For this review, take the finished solid that the model builds, in its own axes (mm). Coordinates: 2 decimals unless noted, no trailing zeros. Order: outer loops, then holes, each group sorted by start corner. A loop starts at its lowest first (then second) coordinate and runs counter-clockwise, first axis right, second up. Notation, with made-up numbers: (-2, -12) -> (51, -12) arc R13 ccw to (51, 8) -> close; hole circle Ø8 at (3.5, 57). An arc over 180 degrees is marked (long way). Write item = value, one per line. Start each with the question number.
1) Insertion check: pin 1 Ø6.5 at (x, z) = (0, 666.75) entering from -Y; pin 2 Ø3 at (y, z) = (5, -249.5) entering from -X; pin 3 Ø5 at (x, z) = (0, 30) entering from -Y; pin 4 Ø5 at (x, z) = (-7.5, -343.5) entering from -Y. Each pin has a flat end and moves straight along its axis. Give the tip position at first contact, or say it passes through.
2) Wall thickness on probe 1 along Z at (x, y) = (0, -12.05); probe 2 along Y at (x, z) = (1.75, 98.5); probe 3 along X at (y, z) = (-2, 296): over which ranges is each line inside the solid? List them lowest first. Write a range as [from, to].
3) Consider section A-A on y = 0. Give the boundary of the cut face in (x, z), and give its area (3 significant figures).
4) Consider section B-B on z = -119. Give the boundary of the cut face in (x, y) (1 decimal), and give its area (3 significant figures).
from build123d import *

# Parameters (mm, degrees)
SKETCH1_R                                  = 12.7
SKETCH1_R_2                                = 11.1125
BOSS_EXTRUDE1_DEPTH                        = 716.7546056
M5_CLEARANCE_HOLE1_D                       = 5.5
SKETCH7_W                                  = 2.75
SKETCH7_H                                  = 12.7
MIRROR1_AT_THE_SECOND_PLANE_COPY_1_SKETC_W = 2.75
MIRROR1_AT_THE_SECOND_PLANE_COPY_1_SKETC_H = 12.7
CUT_EXTRUDE1_START                         = -12.7
SKETCH8_R                                  = 2.5
CUT_EXTRUDE1_DEPTH                         = 25.4


with BuildPart() as part:
    # Sketch1 → Boss-Extrude1 (new body, symmetric)
    with BuildSketch(Plane.XY):
        Circle(SKETCH1_R)
        Circle(SKETCH1_R_2, mode=Mode.SUBTRACT)
    extrude(amount=BOSS_EXTRUDE1_DEPTH, both=True)

    # M5 Clearance Hole1 (through all)
    with Locations(Plane(origin=(0, 12.7, 0), x_dir=(1, 0, 0), z_dir=(0, 1, 0))):
        with Locations((0, 30), (0, -30)):
            Hole(M5_CLEARANCE_HOLE1_D / 2)

    # Sketch7 → M5 Clearance Hole2 (revolve, cut)
    with BuildSketch(Plane(origin=(0, 0, 666.7546056), x_dir=(0, 0, -1), z_dir=(1, 0, 0))):
        with Locations((1.375, 6.35)):
            Rectangle(SKETCH7_W, SKETCH7_H)
    m5_clearance_hole2 = revolve(axis=Axis((0, -6.35, 666.7546056), (0, 1, 0)), mode=Mode.SUBTRACT)

    # Mirror1: M5 Clearance Hole2 across plane
    add(m5_clearance_hole2.mirror(Plane.ZX), mode=Mode.SUBTRACT)

    # Mirror1 at the second plane: M5 Clearance Hole2 across plane
    add(m5_clearance_hole2.mirror(Plane.XY), mode=Mode.SUBTRACT)

    # Mirror1 at the second plane copy 1 sketc → Mirror1 at the second plane copy 1 (revolve, cut)
    with BuildSketch(Plane(origin=(0, 0, -666.7546056), x_dir=(0, 0, 1), z_dir=(1, 0, 0))):
        with Locations((1.375, 6.35)):
            Rectangle(MIRROR1_AT_THE_SECOND_PLANE_COPY_1_SKETC_W, MIRROR1_AT_THE_SECOND_PLANE_COPY_1_SKETC_H)
    revolve(axis=Axis((0, 6.35, -666.7546056), (0, -1, 0)), mode=Mode.SUBTRACT)

    # Sketch8 → Cut-Extrude1 (cut)
    with BuildSketch(Plane(origin=(0, 0, 0), x_dir=(-0.834407926, -0.55114736, 0), z_dir=(0.55114736, -0.834407926, 0)).offset(CUT_EXTRUDE1_START)):
        with Locations((1.717033262, 267.917598195)):
            Circle(SKETCH8_R)
    cut_extrude1 = extrude(amount=CUT_EXTRUDE1_DEPTH, mode=Mode.SUBTRACT)

    # Mirror2: Cut-Extrude1 across plane
    add(cut_extrude1.mirror(Plane.XY), mode=Mode.SUBTRACT)


solid = part.part
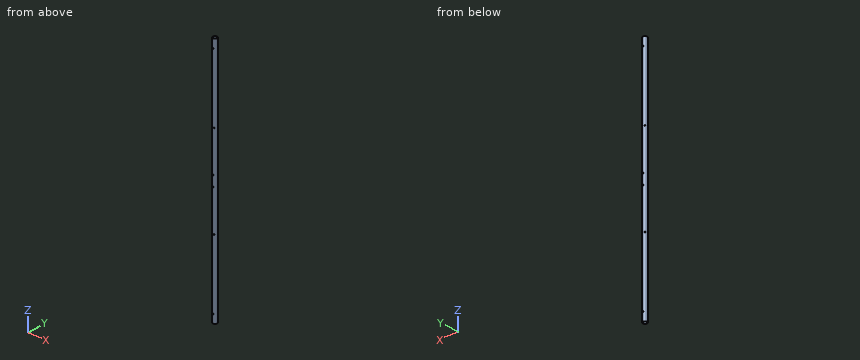
Answer sheet:
q1.pin_1 = -12.7
q1.pin_2 = -12.21
q1.pin_3 = through
q1.pin_4 = -11.67
q2.probe_1 = [-716.75, -669.5], [-664, -32.75], [-27.25, 27.25], [32.75, 664], [669.5, 716.75]
q2.probe_2 = [-12.58, -10.97], [10.97, 12.58]
q2.probe_3 = [-12.54, -10.93], [10.93, 12.54]
q3.outline = (-12.7, -716.75) -> (-11.11, -716.75) -> (-11.11, 716.75) -> (-12.7, 716.75) -> close; (11.11, -716.75) -> (12.7, -716.75) -> (12.7, 716.75) -> (11.11, 716.75) -> close
q3.area = 4,550 mm2
q4.outline = circle Ø25.4 at (0, 0); hole circle Ø22.2 at (0, 0)
q4.area = 119 mm2
